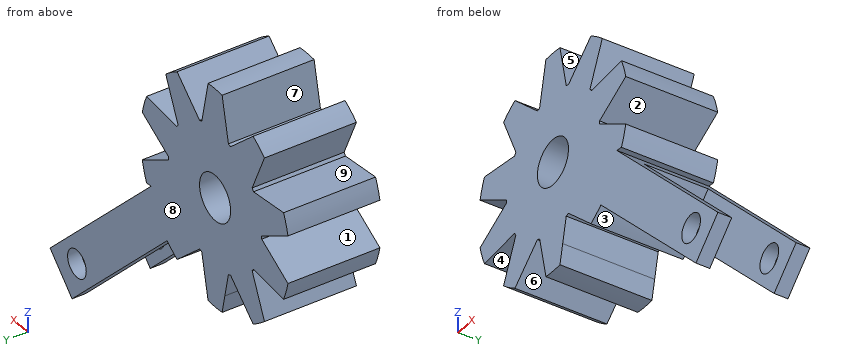
```python
from build123d import *

# Parameters (mm, degrees)
SKETCH1_R           = 2.5
BOSS_EXTRUDE1_DEPTH = 10
BOSS_EXTRUDE2_DEPTH = 10
SKETCH3_R           = 1.5
CUT_EXTRUDE1_DEPTH  = 55
SKETCH4_W           = 40
SKETCH4_H           = 7
CUT_EXTRUDE2_DEPTH  = 10


with BuildPart() as part:
    # Sketch1 → Boss-Extrude1 (new body)
    # profile 1 of 2: a face of its own
    with BuildSketch(Plane(origin=(0, 0, 0), x_dir=(1, 0, 0), z_dir=(0, 1, 0))):
        with BuildLine():
            Line((1.57, 9.875986027), (-1.57, 9.875986027))
            Line((-1.57, 9.875986027), (-2.141392001, 7.187798015))
            ThreePointArc((-2.141392001, 7.187798015), (-2.317627458, 7.132923872), (-2.492459149, 7.073729383))
            Line((-2.492459149, 7.073729383), (-6.108014237, 10.329189807))
            ThreePointArc((-6.108014237, 10.329189807), (-7.053423028, 9.708203932), (-7.936163073, 9.000961931))
            Line((-7.936163073, 9.000961931), (-5.95730419, 4.556372108))
            ThreePointArc((-5.95730419, 4.556372108), (-6.067627458, 4.408389392), (-6.17427562, 4.257736555))
            Line((-6.17427562, 4.257736555), (-11.012832757, 4.766289403))
            ThreePointArc((-11.012832757, 4.766289403), (-11.412678196, 3.708203932), (-11.711123476, 2.617171553))
            Line((-11.711123476, 2.617171553), (-7.497728659, 0.184566922))
            ThreePointArc((-7.497728659, 0.184566922), (-7.5, 0), (-7.497728659, -0.184566922))
            Line((-7.497728659, -0.184566922), (-11.711123476, -2.617171553))
            ThreePointArc((-11.711123476, -2.617171553), (-11.412678196, -3.708203932), (-11.012832757, -4.766289403))
            Line((-11.012832757, -4.766289403), (-6.17427562, -4.257736555))
            ThreePointArc((-6.17427562, -4.257736555), (-6.067627458, -4.408389392), (-5.95730419, -4.556372108))
            Line((-5.95730419, -4.556372108), (-7.936163073, -9.000961931))
            ThreePointArc((-7.936163073, -9.000961931), (-7.053423028, -9.708203932), (-6.108014237, -10.329189807))
            Line((-6.108014237, -10.329189807), (-2.492459149, -7.073729383))
            ThreePointArc((-2.492459149, -7.073729383), (-2.317627458, -7.132923872), (-2.141392001, -7.187798015))
            Line((-2.141392001, -7.187798015), (-1.129858117, -11.946690782))
            ThreePointArc((-1.129858117, -11.946690782), (0, -12), (1.129858117, -11.946690782))
            Line((1.129858117, -11.946690782), (2.141392001, -7.187798015))
            ThreePointArc((2.141392001, -7.187798015), (2.317627458, -7.132923872), (2.492459149, -7.073729383))
            Line((2.492459149, -7.073729383), (6.108014237, -10.329189807))
            ThreePointArc((6.108014237, -10.329189807), (7.053423028, -9.708203932), (7.936163073, -9.000961931))
            Line((7.936163073, -9.000961931), (5.95730419, -4.556372108))
            ThreePointArc((5.95730419, -4.556372108), (6.067627458, -4.408389392), (6.17427562, -4.257736555))
            Line((6.17427562, -4.257736555), (11.012832757, -4.766289403))
            ThreePointArc((11.012832757, -4.766289403), (11.412678196, -3.708203932), (11.711123476, -2.617171553))
            Line((11.711123476, -2.617171553), (7.497728659, -0.184566922))
            ThreePointArc((7.497728659, -0.184566922), (7.5, 0), (7.497728659, 0.184566922))
            Line((7.497728659, 0.184566922), (11.711123476, 2.617171553))
            ThreePointArc((11.711123476, 2.617171553), (11.412678196, 3.708203932), (11.012832757, 4.766289403))
            Line((11.012832757, 4.766289403), (6.17427562, 4.257736555))
            ThreePointArc((6.17427562, 4.257736555), (6.067627458, 4.408389392), (5.95730419, 4.556372108))
            Line((5.95730419, 4.556372108), (7.936163073, 9.000961931))
            ThreePointArc((7.936163073, 9.000961931), (7.053423028, 9.708203932), (6.108014237, 10.329189807))
            Line((6.108014237, 10.329189807), (2.492459149, 7.073729383))
            ThreePointArc((2.492459149, 7.073729383), (2.317627458, 7.132923872), (2.141392001, 7.187798015))
            Line((2.141392001, 7.187798015), (1.57, 9.875986027))
        make_face()
        with Locations(Location((0, 0, 0), (0, 0, 270))):
            Circle(SKETCH1_R, mode=Mode.SUBTRACT)
    # profile 2 of 2: a face of its own
    with BuildSketch(Plane(origin=(0, 0, 0), x_dir=(1, 0, 0), z_dir=(0, 1, 0))):
        with BuildLine():
            Line((-1.129858117, 11.946690782), (-1.57, 9.875986027))
            Line((-1.57, 9.875986027), (1.57, 9.875986027))
            Line((1.57, 9.875986027), (1.129858117, 11.946690782))
            ThreePointArc((1.129858117, 11.946690782), (0, 12), (-1.129858117, 11.946690782))
        make_face()
    extrude(amount=BOSS_EXTRUDE1_DEPTH)

    # Sketch2 → Boss-Extrude2 (add)
    with BuildSketch(Plane(origin=(0, 10, 0), x_dir=(1, 0, 0), z_dir=(0, 1, 0))):
        Polygon((1.781492434, 3.263264717), (22.99469587, 24.476468153), (26.530229776, 20.940934247), (5.31702634, -0.272269189), align=None)
    extrude(amount=-BOSS_EXTRUDE2_DEPTH)

    # Sketch3 → Cut-Extrude1 (cut)
    with BuildSketch(Plane(origin=(0, 10, 0), x_dir=(1, 0, 0), z_dir=(0, 1, 0))):
        with Locations(Location((22.215215239, 20.161453616, 0), (0, 0, 270))):
            Circle(SKETCH3_R)
    extrude(amount=-CUT_EXTRUDE1_DEPTH, mode=Mode.SUBTRACT)

    # Sketch4 → Cut-Extrude2 (cut)
    with BuildSketch(Plane(origin=(2.794647764, 0, 2.794647764), x_dir=(0.7071067811865461, 0, -0.707106781186549), z_dir=(0.707106781186549, 0, 0.7071067811865461))):
        with Locations((33.567181991, 5)):
            Rectangle(SKETCH4_W, SKETCH4_H)
    extrude(amount=-CUT_EXTRUDE2_DEPTH, mode=Mode.SUBTRACT)


solid = part.part
```
Source: CAD feature listing. Evaluate the final solid. Frame: model axes, mm. Face numbers are marked on the shaded views. A direction names the side the tool comes from. Coordinates: 2 decimals unless noted, no trailing zeros. Write each loop counter-clockwise with the first axis right and the second up, starting at its lowest first coordinate (ties: lowest second). Pieces come first, ordered by that corner, then holes. Notation, with made-up numbers: M 0,87.25 L 23,87.25 A19 cw 23,106.25 Z; hole C 49.5,51.5 d8. An arc over 180 degrees is marked long. Answer as a JSON object with one key per item and string values.
1. Draft query along Z for the marked faces 6, 7, 8 and 9. Return one class per face: released by +Z, released by -Z, zero draft, split by the parting line, or undercut.
Evaluation:
{"face 6": "released by -Z", "face 7": "released by +Z", "face 8": "zero draft", "face 9": "undercut"}
2. Cut plane D-D on x = -4.5. Output: boundary loops of the cut face in (y, z).
Evaluation:
{"outline": "M 0,-8.88 L 10,-8.88 L 10,8.88 L 0,8.88 Z"}
3. Cut plane C-C on z = -6. Output: boundary loops of the cut face in (x, y), plus the area to 3 significant figures.
Evaluation:
{"outline": "M -6.6,0 L 11.59,0 L 11.59,10 L -6.6,10 Z", "area": "182 mm^2"}
4. Ray query, L1, parallel to Y at x = 15.5, z = -12.5; L2, parallel to X at y = 4, z = 0; L3, parallel to X at y = 2.5, z = -1. Return the intervals inside material, ascending.
Evaluation:
{"L1": "0 to 1.5, 8.5 to 10", "L2": "-7.5 to -2.5, 2.5 to 7.5", "L3": "-8.91 to -2.29, 2.29 to 8.91"}
5. Contact query for flat-ended pins moving along their axis: P1, Ø5, axis at x = 10.5, z = 7, coming from the -Y side; P2, Ø4, axis at y = 1.5, z = 6, coming from the -X side; P3, Ø10, axis at x = 1, z = -17.5, coming from the -Y side; P4, Ø6, axis at y = 8.5, z = -14.5, coming from the -X side. Output: stop coordinate, or through.
Evaluation:
{"P1": "y = 0", "P2": "x = -11.31", "P3": "through", "P4": "x = -1.22"}
6. Cut plane A-A on x = 0. Output: boundary loops of the cut face in (y, z), plus the area to 3 significant figures.
Evaluation:
{"outline": "M 0,-12 L 10,-12 L 10,-2.5 L 0,-2.5 Z; M 0,2.5 L 10,2.5 L 10,12 L 0,12 Z", "area": "190 mm^2"}
7. Access query for the marked faces 1, 2, 3, 4 and 5. Directions: +Z, -Z, +X, -X, +Y, -Y. A direction counts if a zero-diameter tool reaches every point of the face in a straight line with its end or side. Return the directions, or none.
Evaluation:
{"face 1": "-X, +Y, -Y", "face 2": "+X, +Y, -Y", "face 3": "-Z, +Y, -Y", "face 4": "+Y, -Y", "face 5": "+Z, +Y, -Y"}
8. Cut plane B-B on z = 2. Output: boundary loops of the cut face in (x, y).
Evaluation:
{"outline": "M -10.64,0 L -1.5,0 L -1.5,10 L -10.64,10 Z; M 1.5,0 L 10.64,0 L 10.64,10 L 1.5,10 Z"}
